from build123d import *

# Parameters (mm, degrees)
SK_KNEE_PLATE_R         = 2.75
SK_KNEE_PLATE_R_2       = 6
KNEE_PLATE_DEPTH        = 8
SK_KNEE_PILOT_RECESS_R  = 25.15
KNEE_PILOT_RECESS_DEPTH = 2.2
SK_JOGGLE_W             = 68
SK_JOGGLE_H             = 33
JOGGLE_DEPTH            = 18
SK_WEB_R                = 1.7
SK_WEB_R_2              = 11
SK_WEB_R_3              = 8
WEB_DEPTH               = 10
SK_FORK_BAR_W           = 60
SK_FORK_BAR_H           = 54
FORK_BAR_DEPTH          = 10
SK_TINE_LAT_R           = 4
TINE_LAT_DEPTH          = 9
SK_TINE_MED_R           = 4
TINE_MED_DEPTH          = 9


with BuildPart() as part:
    # SK_Knee_Plate → Knee_Plate (new body)
    with BuildSketch(Plane(origin=(0, 20, 0), x_dir=(1, 0, 0), z_dir=(0, 1, 0))):
        Polygon((-34, -40), (34, -40), (44, 0), (36, 84), (-36, 84), (-44, 0), align=None)
        with Locations(Location((29.56414504, 12.245869836, 0), (0, 0, 270))):
            Circle(SK_KNEE_PLATE_R, mode=Mode.SUBTRACT)
        with Locations(Location((12.245869836, 29.56414504, 0), (0, 0, 270))):
            Circle(SK_KNEE_PLATE_R, mode=Mode.SUBTRACT)
        with Locations(Location((-12.245869836, 29.56414504, 0), (0, 0, 270))):
            Circle(SK_KNEE_PLATE_R, mode=Mode.SUBTRACT)
        with Locations(Location((-29.56414504, 12.245869836, 0), (0, 0, 270))):
            Circle(SK_KNEE_PLATE_R, mode=Mode.SUBTRACT)
        with Locations(Location((-29.56414504, -12.245869836, 0), (0, 0, 270))):
            Circle(SK_KNEE_PLATE_R, mode=Mode.SUBTRACT)
        with Locations(Location((-12.245869836, -29.56414504, 0), (0, 0, 270))):
            Circle(SK_KNEE_PLATE_R, mode=Mode.SUBTRACT)
        with Locations(Location((12.245869836, -29.56414504, 0), (0, 0, 270))):
            Circle(SK_KNEE_PLATE_R, mode=Mode.SUBTRACT)
        with Locations(Location((29.56414504, -12.245869836, 0), (0, 0, 270))):
            Circle(SK_KNEE_PLATE_R, mode=Mode.SUBTRACT)
        with Locations(Location((0, 0, 0), (0, 0, 270))):
            Circle(SK_KNEE_PLATE_R_2, mode=Mode.SUBTRACT)
    extrude(amount=KNEE_PLATE_DEPTH)

    # SK_Knee_Pilot_Recess → Knee_Pilot_Recess (cut)
    with BuildSketch(Plane(origin=(0, 20, 0), x_dir=(1, 0, 0), z_dir=(0, 1, 0))):
        with Locations(Location((0, 0, 0), (0, 0, 270))):
            Circle(SK_KNEE_PILOT_RECESS_R)
    extrude(amount=KNEE_PILOT_RECESS_DEPTH, mode=Mode.SUBTRACT)

    # SK_Joggle → Joggle (add)
    with BuildSketch(Plane.XY.offset(-84)):
        with Locations((0, 11.5)):
            Rectangle(SK_JOGGLE_W, SK_JOGGLE_H)
    extrude(amount=JOGGLE_DEPTH)

    # SK_Web → Web (add)
    with BuildSketch(Plane(origin=(0, -5, 0), x_dir=(1, 0, 0), z_dir=(0, 1, 0))):
        Polygon((-34, 66), (34, 66), (48, 88), (48, 236), (30, 264), (-30, 264), (-48, 236), (-48, 88), align=None)
        with Locations(Location((37, 118, 0), (0, 0, 270))):
            Circle(SK_WEB_R, mode=Mode.SUBTRACT)
        with Locations(Location((18.5, 150.04293994, 0), (0, 0, 270))):
            Circle(SK_WEB_R, mode=Mode.SUBTRACT)
        with Locations(Location((-18.5, 150.04293994, 0), (0, 0, 270))):
            Circle(SK_WEB_R, mode=Mode.SUBTRACT)
        with Locations(Location((-37, 118, 0), (0, 0, 270))):
            Circle(SK_WEB_R, mode=Mode.SUBTRACT)
        with Locations(Location((-18.5, 85.95706006, 0), (0, 0, 270))):
            Circle(SK_WEB_R, mode=Mode.SUBTRACT)
        with Locations(Location((18.5, 85.95706006, 0), (0, 0, 270))):
            Circle(SK_WEB_R, mode=Mode.SUBTRACT)
        with Locations(Location((37, 206, 0), (0, 0, 270))):
            Circle(SK_WEB_R, mode=Mode.SUBTRACT)
        with Locations(Location((18.5, 238.04293994, 0), (0, 0, 270))):
            Circle(SK_WEB_R, mode=Mode.SUBTRACT)
        with Locations(Location((-18.5, 238.04293994, 0), (0, 0, 270))):
            Circle(SK_WEB_R, mode=Mode.SUBTRACT)
        with Locations(Location((-37, 206, 0), (0, 0, 270))):
            Circle(SK_WEB_R, mode=Mode.SUBTRACT)
        with Locations(Location((-18.5, 173.95706006, 0), (0, 0, 270))):
            Circle(SK_WEB_R, mode=Mode.SUBTRACT)
        with Locations(Location((18.5, 173.95706006, 0), (0, 0, 270))):
            Circle(SK_WEB_R, mode=Mode.SUBTRACT)
        with Locations(Location((0, 118, 0), (0, 0, 270))):
            Circle(SK_WEB_R_2, mode=Mode.SUBTRACT)
        with Locations(Location((0, 206, 0), (0, 0, 270))):
            Circle(SK_WEB_R_2, mode=Mode.SUBTRACT)
        with Locations(Location((0, 162, 0), (0, 0, 270))):
            Circle(SK_WEB_R_3, mode=Mode.SUBTRACT)
    extrude(amount=WEB_DEPTH)

    # SK_Fork_Bar → Fork_Bar (add)
    with BuildSketch(Plane.XY.offset(-270)):
        Rectangle(SK_FORK_BAR_W, SK_FORK_BAR_H)
    extrude(amount=FORK_BAR_DEPTH)

    # SK_Tine_Lat → Tine_Lat (add)
    with BuildSketch(Plane(origin=(0, -27, 0), x_dir=(1, 0, 0), z_dir=(0, 1, 0))):
        Polygon((-16, 260), (16, 260), (16, 308), (8, 318), (-8, 318), (-16, 308), align=None)
        with Locations(Location((0, 300, 0), (0, 0, 270))):
            Circle(SK_TINE_LAT_R, mode=Mode.SUBTRACT)
    extrude(amount=TINE_LAT_DEPTH)

    # SK_Tine_Med → Tine_Med (add)
    with BuildSketch(Plane(origin=(0, 18, 0), x_dir=(1, 0, 0), z_dir=(0, 1, 0))):
        Polygon((-16, 260), (16, 260), (16, 308), (8, 318), (-8, 318), (-16, 308), align=None)
        with Locations(Location((0, 300, 0), (0, 0, 270))):
            Circle(SK_TINE_MED_R, mode=Mode.SUBTRACT)
    extrude(amount=TINE_MED_DEPTH)


solid = part.part
Here's how the part is built. I have some questions about the finished solid (model axes, mm). A direction names the side the tool comes from. Coordinates: 2 decimals unless noted, no trailing zeros. Write each loop counter-clockwise with the first axis right and the second up, starting at its lowest first coordinate (ties: lowest second). Pieces come first, ordered by that corner, then holes.
Item 1: If I drill on line 1 (Z direction, x = -18, y = -1); line 2 (X direction, y = 1.5, z = -118); line 3 (X direction, y = 24.15, z = 0), over which ranges is the centre line in solid material (lowest first)?
Item 2: If we mould it in two halves opening along Z, with no side actions, what happens to faces 1 (the flat face through (-5, 22.2, 5)), 2 (the flat face through (39, 0, -250)), 3 (the cylindrical face through (-15.3, 21.08, -19.96)), 4 (the flat face through (16, 22, -289))? For each: +Z half, -Z half, draft (parallel to the pull), parting line (faces both ways), or undercut.
Item 3: I want a section at B-B on y = 10. Write out the boundary of the cut face in (x, z).
Item 4: I want a section at A-A on z = -162. Write out the boundary of the cut face in (x, y).
Item 5: Will these pins go through, and if not, where does the flat tip stop? pin 1 (16 mm diameter, centred on x = 11, y = -5, fed in from -Z); pin 2 (1 mm diameter, centred on x = 36.5, z = -140, fed in from -Y); pin 3 (2.5 mm diameter, centred on y = 24.5, z = -288.5, fed in from +X).
Item 6: On a 3-axis mill with a long thin cutter (end or side, diameter ignored), from which of +Z, -Z, +X, -X, +Y, -Y can I reach the whole of each face in a straight line? I mean faces 5 (the flat face through (0, 27, -283)), 6 (the flat face through (0, 18, -294)), 7 (the flat face through (0, 16, -260)), 8 (the flat face through (-34, 12, -75)), 9 (the flat face through (30, 0, -265)). Say none if no direction works.
Item 7: I want a section at C-C on z = -300. Write out the boundary of the cut face in (x, y).
Item 8: I want a section at D-D on x = 0. Count the separate pieces of the cut face and the enclosed holes in it, and give its area (3 significant figures).
Findings below:
1. line 1: z = -270 to -239.67, -236.42 to -175.58, -172.33 to -151.67, -148.42 to -87.58, -84.33 to -66
1. line 2: x = -48 to -38.7, -35.3 to -11, 11 to 35.3, 38.7 to 48
1. line 3: x = -44 to -6, 6 to 44
2. face 1: undercut
2. face 2: -Z half
2. face 3: undercut
2. face 4: draft
3. outline: (-34, -84) - (34, -84) - (34, -66) - (-34, -66) - close; (-30, -270) - (30, -270) - (30, -260) - (-30, -260) - close
4. outline: (-48, -5) - (-8, -5) - (-8, 5) - (-48, 5) - close; (8, -5) - (48, -5) - (48, 5) - (8, 5) - close
5. pin 1: stops at z = -270
5. pin 2: stops at y = -5
5. pin 3: stops at x = 16
6. face 5: -Z, +X, -X, +Y
6. face 6: -Z, +X, -X
6. face 7: +X, -X, +Y
6. face 8: +Z, -Z, -X
6. face 9: -Z, +X
7. outline: (-16, -27) - (-4, -27) - (-4, -18) - (-16, -18) - close; (-16, 18) - (-4, 18) - (-4, 27) - (-16, 27) - close; (4, -27) - (16, -27) - (16, -18) - (4, -18) - close; (4, 18) - (16, 18) - (16, 27) - (4, 27) - close
8. separate pieces: 7
8. enclosed holes: 0
8. area: 3,680 mm2
